Work out the finished part from the listing and answer in its coordinate system (mm). A direction names the side the tool comes from. Coordinates: 2 decimals unless noted, no trailing zeros. Order: outer loops, then holes, each group sorted by start corner. A loop starts at its lowest first (then second) coordinate and runs counter-clockwise, first axis right, second up.
1. The part is cut by section B-B, the plane y = 11.5. Give the vertices of the cut face in (x, z).
2. A tool of negligible diameter and unlimited length cuts with its end or side. For faces 4 (the flat face through (-13, 20, -13)), 5 (the flat face through (-13, -20, -13)), 6 (the flat face through (0, 0, -20)), 7 (the cylindrical face through (-13.55, -5.78, -7.54)), 8 (the flat face through (0, 0, 20)), from which of +Z, -Z, +X, -X, +Y, -Y can it reach the whole face along a straight path? Write none if from no direction.
3. Flat-ended cylindrical pins translate along their axes: pin 1 Ø1 at (x, y) = (4, -49.5) entering from +Z; pin 2 Ø22.5 at (x, z) = (0, 0) entering from -Y; pin 3 Ø1 at (x, z) = (10, -3) entering from +Y; pin 4 Ø1.5 at (x, y) = (-8, -48.5) entering from -Z. Find the tip coordinate at first contact, or state that the pin passes through.
4. The part is cut by section D-D, the plane y = 0. Give the vertices of the cut face in (x, z).
5. The part is cut by section C-C, the plane z = 0. Count the separate pieces of the cut face and the enclosed holes in it, then the cut area to 3 significant figures.
6. Determine the mould class of faces 1 (the cylindrical face through (-5.407, 29.633, -17.169)), 2 (the flat face through (-13, 40, 6)), 3 (the flat face through (10, 22, -3)) for opening direction X: +X half, -X half, draft (parallel to the pull), parting line (faces both ways), or undercut.
7. Find the intervals of material crossed by probe 1 along Y at (x, z) = (-3.5, 13); probe 2 along X at (y, z) = (-43, 0); probe 3 along Z at (x, y) = (4, -8), in increasing order.
```python
from build123d import *

# Parameters (mm, degrees)
CROQUIS1_W              = 40
CROQUIS1_H              = 40
SALIENTE_EXTRUIR2_DEPTH = 20
CROQUIS4_R              = 18
SALIENTE_EXTRUIR3_DEPTH = 40
REDONDEO1_R             = 1
CROQUIS5_R              = 16
SALIENTE_EXTRUIR4_DEPTH = 20
REDONDEO2_R             = 1
CROQUIS6_R              = 14
CORTAR_EXTRUIR1_DEPTH   = 18
CROQUIS7_R              = 10
CORTAR_EXTRUIR3_DEPTH   = 104.923048454
CROQUIS8_R              = 9.5
CORTAR_EXTRUIR4_DEPTH   = 18
REDONDEO3_R             = 1


with BuildPart() as part:
    # Croquis1 → Saliente-Extruir2 (new, symmetric)
    with BuildSketch(Plane(origin=(0, 0, 0), x_dir=(1, 0, 0), z_dir=(0, 1, 0))):
        Rectangle(CROQUIS1_W, CROQUIS1_H)
    extrude(amount=SALIENTE_EXTRUIR2_DEPTH, both=True)

    # Croquis4 → Saliente-Extruir3 (add, symmetric)
    with BuildSketch(Plane(origin=(0, 0, 0), x_dir=(1, 0, 0), z_dir=(0, 1, 0))):
        with Locations(Location((0, 0, 0), (0, 0, 90))):
            Circle(CROQUIS4_R)
    extrude(amount=SALIENTE_EXTRUIR3_DEPTH, both=True)

    # Redondeo1
    redondeo1_edges = [part.edges().sort_by_distance(p)[0] for p in [
        (-20, 20, 0),
        (0, 20, 20),
        (0, -40, 18),
        (0, 40, 18),
        (20, 20, 0),
        (0, -20, 20),
        (-20, -20, 0),
        (0, -20, -20),
        (20, -20, 0),
        (0, 20, -20),
    ]]
    fillet(redondeo1_edges, radius=REDONDEO1_R)

    # Croquis5 → Saliente-Extruir4 (add)
    with BuildSketch(Plane.XZ.offset(40)):
        with Locations(Location((0, 0, 0), (0, 0, 90))):
            Circle(CROQUIS5_R)
    extrude(amount=SALIENTE_EXTRUIR4_DEPTH)

    # Redondeo2
    redondeo2_edges = [part.edges().sort_by_distance(p)[0] for p in [
        (0, -60, -16),
    ]]
    fillet(redondeo2_edges, radius=REDONDEO2_R)

    # Croquis6 → Cortar-Extruir1 (cut)
    with BuildSketch(Plane(origin=(0, 40, 0), x_dir=(1, 0, 0), z_dir=(0, 1, 0))):
        with Locations(Location((0, 0, 0), (0, 0, 270))):
            Circle(CROQUIS6_R)
    extrude(amount=-CORTAR_EXTRUIR1_DEPTH, mode=Mode.SUBTRACT)

    # Croquis7 → Cortar-Extruir3 (cut, through all)
    with BuildSketch(Plane.XZ.offset(60)):
        with Locations(Location((0, 0, 0), (0, 0, 270))):
            Circle(CROQUIS7_R)
    extrude(amount=-CORTAR_EXTRUIR3_DEPTH, mode=Mode.SUBTRACT)

    # Croquis8 → Cortar-Extruir4 (cut)
    with BuildSketch(Plane.ZY.offset(20)):
        Circle(CROQUIS8_R)
    extrude(amount=-CORTAR_EXTRUIR4_DEPTH, mode=Mode.SUBTRACT)

    # Redondeo3
    # the kernel refuses this fillet: 1 mm, written as the material it takes off along each edge
    with BuildSketch(Plane(origin=(19, -19, 19), x_dir=(1, 0, 0), z_dir=(0, 0, 1))) as redondeo3_piece_1_section:
        Polygon((0, 0), (REDONDEO3_R, 0), (REDONDEO3_R, -REDONDEO3_R), (0, -REDONDEO3_R), align=None)
    redondeo3_piece_1 = extrude(amount=REDONDEO3_R, mode=Mode.PRIVATE)
    redondeo3_piece_1 = redondeo3_piece_1 - Plane(origin=(19, -19, 19), x_dir=(-0.7071067811865475, 0.7071067811865475, 0), z_dir=(0, 0, 1)) * Sphere(REDONDEO3_R, mode=Mode.PRIVATE)
    add(redondeo3_piece_1, mode=Mode.SUBTRACT)
    with BuildSketch(Plane(origin=(-19, -19, 19), x_dir=(0, 0, 1), z_dir=(-1, 0, 0))) as redondeo3_piece_2_section:
        Polygon((0, 0), (REDONDEO3_R, 0), (REDONDEO3_R, -REDONDEO3_R), (0, -REDONDEO3_R), align=None)
    redondeo3_piece_2 = extrude(amount=REDONDEO3_R, mode=Mode.PRIVATE)
    redondeo3_piece_2 = redondeo3_piece_2 - Plane(origin=(-19, -19, 19), x_dir=(0, 0.7071067811865475, -0.7071067811865475), z_dir=(-1, 0, 0)) * Sphere(REDONDEO3_R, mode=Mode.PRIVATE)
    add(redondeo3_piece_2, mode=Mode.SUBTRACT)
    with BuildSketch(Plane(origin=(19, -19, -19), x_dir=(1, 0, 0), z_dir=(0, 0, -1))) as redondeo3_piece_3_section:
        Polygon((0, 0), (REDONDEO3_R, 0), (REDONDEO3_R, REDONDEO3_R), (0, REDONDEO3_R), align=None)
    redondeo3_piece_3 = extrude(amount=REDONDEO3_R, mode=Mode.PRIVATE)
    redondeo3_piece_3 = redondeo3_piece_3 - Plane(origin=(19, -19, -19), x_dir=(-0.7071067811865475, 0.7071067811865475, 0), z_dir=(0, 0, -1)) * Sphere(REDONDEO3_R, mode=Mode.PRIVATE)
    add(redondeo3_piece_3, mode=Mode.SUBTRACT)
    with BuildSketch(Plane(origin=(-19, -19, -19), x_dir=(0, 0, -1), z_dir=(-1, 0, 0))) as redondeo3_piece_4_section:
        Polygon((0, 0), (REDONDEO3_R, 0), (REDONDEO3_R, REDONDEO3_R), (0, REDONDEO3_R), align=None)
    redondeo3_piece_4 = extrude(amount=REDONDEO3_R, mode=Mode.PRIVATE)
    redondeo3_piece_4 = redondeo3_piece_4 - Plane(origin=(-19, -19, -19), x_dir=(0, 0.7071067811865475, 0.7071067811865475), z_dir=(-1, 0, 0)) * Sphere(REDONDEO3_R, mode=Mode.PRIVATE)
    add(redondeo3_piece_4, mode=Mode.SUBTRACT)
    with BuildSketch(Plane(origin=(19, 19, 19), x_dir=(1, 0, 0), z_dir=(0, 0, 1))) as redondeo3_piece_5_section:
        Polygon((0, 0), (REDONDEO3_R, 0), (REDONDEO3_R, REDONDEO3_R), (0, REDONDEO3_R), align=None)
    redondeo3_piece_5 = extrude(amount=REDONDEO3_R, mode=Mode.PRIVATE)
    redondeo3_piece_5 = redondeo3_piece_5 - Plane(origin=(19, 19, 19), x_dir=(-0.7071067811865475, -0.7071067811865475, 0), z_dir=(0, 0, 1)) * Sphere(REDONDEO3_R, mode=Mode.PRIVATE)
    add(redondeo3_piece_5, mode=Mode.SUBTRACT)
    with BuildSketch(Plane(origin=(-19, 19, 19), x_dir=(0, 0, 1), z_dir=(-1, 0, 0))) as redondeo3_piece_6_section:
        Polygon((0, 0), (REDONDEO3_R, 0), (REDONDEO3_R, REDONDEO3_R), (0, REDONDEO3_R), align=None)
    redondeo3_piece_6 = extrude(amount=REDONDEO3_R, mode=Mode.PRIVATE)
    redondeo3_piece_6 = redondeo3_piece_6 - Plane(origin=(-19, 19, 19), x_dir=(0, -0.7071067811865475, -0.7071067811865475), z_dir=(-1, 0, 0)) * Sphere(REDONDEO3_R, mode=Mode.PRIVATE)
    add(redondeo3_piece_6, mode=Mode.SUBTRACT)
    with BuildSketch(Plane(origin=(19, 19, -19), x_dir=(1, 0, 0), z_dir=(0, 0, -1))) as redondeo3_piece_7_section:
        Polygon((0, 0), (REDONDEO3_R, 0), (REDONDEO3_R, -REDONDEO3_R), (0, -REDONDEO3_R), align=None)
    redondeo3_piece_7 = extrude(amount=REDONDEO3_R, mode=Mode.PRIVATE)
    redondeo3_piece_7 = redondeo3_piece_7 - Plane(origin=(19, 19, -19), x_dir=(-0.7071067811865475, -0.7071067811865475, 0), z_dir=(0, 0, -1)) * Sphere(REDONDEO3_R, mode=Mode.PRIVATE)
    add(redondeo3_piece_7, mode=Mode.SUBTRACT)
    with BuildSketch(Plane(origin=(-19, 19, -19), x_dir=(0, 0, -1), z_dir=(-1, 0, 0))) as redondeo3_piece_8_section:
        Polygon((0, 0), (REDONDEO3_R, 0), (REDONDEO3_R, -REDONDEO3_R), (0, -REDONDEO3_R), align=None)
    redondeo3_piece_8 = extrude(amount=REDONDEO3_R, mode=Mode.PRIVATE)
    redondeo3_piece_8 = redondeo3_piece_8 - Plane(origin=(-19, 19, -19), x_dir=(0, -0.7071067811865475, 0.7071067811865475), z_dir=(-1, 0, 0)) * Sphere(REDONDEO3_R, mode=Mode.PRIVATE)
    add(redondeo3_piece_8, mode=Mode.SUBTRACT)
    with BuildSketch(Plane(origin=(-20, 19, -20), x_dir=(0, 0, 1), z_dir=(0, -1, 0)), Plane(origin=(20, -19, 20), x_dir=(-1, 0, 0), z_dir=(0, 1, 0))) as redondeo3_piece_9:
        with BuildLine():
            CenterArc((REDONDEO3_R, -REDONDEO3_R), REDONDEO3_R, 90, 90)
            Line((0, -REDONDEO3_R), (0, 0))
            Line((0, 0), (REDONDEO3_R, 0))
        make_face()
    extrude(amount=38, mode=Mode.SUBTRACT)
    with BuildSketch(Plane(origin=(20, -19, -20), x_dir=(-1, 0, 0), z_dir=(0, 1, 0)), Plane(origin=(-20, 19, 20), x_dir=(0, 0, -1), z_dir=(0, -1, 0))) as redondeo3_piece_10:
        with BuildLine():
            CenterArc((REDONDEO3_R, REDONDEO3_R), REDONDEO3_R, 180, 90)
            Line((0, REDONDEO3_R), (0, 0))
            Line((0, 0), (REDONDEO3_R, 0))
        make_face()
    extrude(amount=38, mode=Mode.SUBTRACT)


solid = part.part
```
Geometry says:
1. outline: (-20, -19) arc R1 ccw to (-19, -20) - (19, -20) arc R1 ccw to (20, -19) - (20, 19) arc R1 ccw to (19, 20) - (-19, 20) arc R1 ccw to (-20, 19) - close; hole circle Ø20 at (0, 0)
2. face 4: +Y
2. face 5: -Y
2. face 6: -Z, +X, -X, +Y, -Y
2. face 7: -X
2. face 8: +Z, +X, -X, +Y, -Y
3. pin 1: stops at z = 15.61
3. pin 2: stops at y = -60
3. pin 3: stops at y = 22
3. pin 4: stops at z = -14.26
4. outline: (-20, -19) arc R1 ccw to (-19, -20) - (19, -20) arc R1 ccw to (20, -19) - (20, 19) arc R1 ccw to (19, 20) - (-19, 20) arc R1 ccw to (-20, 19) - (-20, 9.5) - (-3.12, 9.5) arc R10 cw (long way) to (-3.12, -9.5) - (-20, -9.5) - close
5. separate pieces: 3
5. enclosed holes: 0
5. area: 1,340 mm2
6. face 1: parting line
6. face 2: draft
6. face 3: undercut
7. probe 1: y = -60 to 22
7. probe 2: x = -16 to -10, 10 to 16
7. probe 3: z = -20 to -9.17, 9.17 to 20
